Check sheet for the modelled part. Datum: model origin and axes. Units: mm. Face numbers are marked on the shaded views. A direction names the side the tool comes from. Coordinates: 2 decimals unless noted, no trailing zeros. Loops run counter-clockwise (first coordinate to the right, second up) from the corner with the lowest first, then second, coordinate; pieces in that order, holes last. Notation, with made-up numbers: M -28.75,-38.75 L 21.25,-38.75 A22 cw 21.25,-17.75 Z; hole C -29.5,-27.5 d2. An arc over 180 degrees is marked long. Answer in a Markdown table with one row per item. Add a question column.
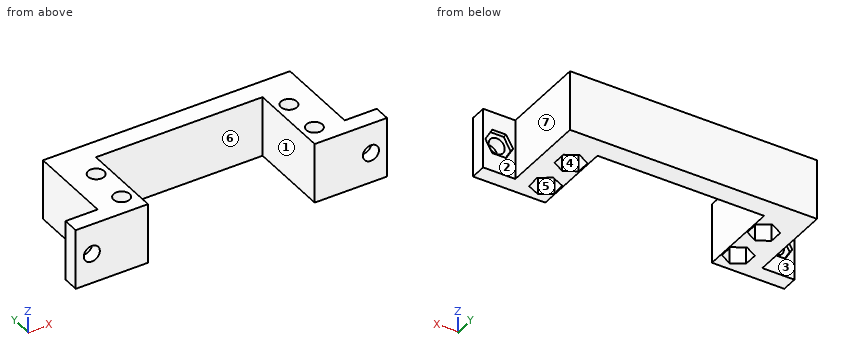
```python
from build123d import *

# Parameters (mm, degrees)
SKETCH1_R           = 2
BOSS_EXTRUDE1_DEPTH = 15
CUT_EXTRUDE1_DEPTH  = 11
CUT_EXTRUDE2_DEPTH  = 1
SKETCH5_R           = 2
CUT_EXTRUDE3_DEPTH  = 4


with BuildPart() as part:
    # Sketch1 → Boss-Extrude1 (new body)
    with BuildSketch(Plane.XY):
        Polygon((0, 0), (0, 20.5), (41.5, 20.5), (41.5, 0), (59.5, 0), (59.5, 4), (51.5, 4), (51.5, 25.5), (-10, 25.5), (-10, 4), (-18, 4), (-18, 0), align=None)
        with Locations((44.75, 5.25)):
            Circle(SKETCH1_R, mode=Mode.SUBTRACT)
        with Locations((44.75, 15.25)):
            Circle(SKETCH1_R, mode=Mode.SUBTRACT)
        with Locations((-3.25, 15.25)):
            Circle(SKETCH1_R, mode=Mode.SUBTRACT)
        with Locations((-3.25, 5.25)):
            Circle(SKETCH1_R, mode=Mode.SUBTRACT)
    extrude(amount=BOSS_EXTRUDE1_DEPTH)

    # Sketch3 → Cut-Extrude1 (cut)
    with BuildSketch(Plane(origin=(0, 0, 0), x_dir=(-1, 0, 0), z_dir=(0, 0, -1))):
        Polygon((3.25, 18.714101615), (0.25, 16.982050808), (0.25, 13.517949192), (3.25, 11.785898385), (6.25, 13.517949192), (6.25, 16.982050808), align=None)
        Polygon((3.25, 8.714101615), (0.25, 6.982050808), (0.25, 3.517949192), (3.25, 1.785898385), (6.25, 3.517949192), (6.25, 6.982050808), align=None)
        Polygon((-44.75, 18.714101615), (-47.75, 16.982050808), (-47.75, 13.517949192), (-44.75, 11.785898385), (-41.75, 13.517949192), (-41.75, 16.982050808), align=None)
        Polygon((-45.037677981, 8.702135771), (-47.883476265, 6.726931446), (-47.595798284, 3.274795675), (-44.462322019, 1.797864229), (-41.616523735, 3.773068554), (-41.904201716, 7.225204325), align=None)
    extrude(amount=-CUT_EXTRUDE1_DEPTH, mode=Mode.SUBTRACT)

    # Sketch4 → Cut-Extrude2 (cut)
    with BuildSketch(Plane(origin=(0, 4, 0), x_dir=(1, 0, 0), z_dir=(0, 1, 0))):
        Polygon((58.964101615, -7.5), (57.232050808, -4.5), (53.767949192, -4.5), (52.035898385, -7.5), (53.767949192, -10.5), (57.232050808, -10.5), align=None)
        Polygon((-17.464101615, -7.5), (-15.732050808, -10.5), (-12.267949192, -10.5), (-10.535898385, -7.5), (-12.267949192, -4.5), (-15.732050808, -4.5), align=None)
    extrude(amount=-CUT_EXTRUDE2_DEPTH, mode=Mode.SUBTRACT)

    # Sketch5 → Cut-Extrude3 (cut)
    with BuildSketch(Plane(origin=(0, 4, 0), x_dir=(1, 0, 0), z_dir=(0, 1, 0))):
        with Locations(Location((55.5, -7.5, 0), (0, 0, 180))):
            Circle(SKETCH5_R)
        with Locations(Location((-14, -7.5, 0), (0, 0, 180))):
            Circle(SKETCH5_R)
    extrude(amount=-CUT_EXTRUDE3_DEPTH, mode=Mode.SUBTRACT)


solid = part.part
```
Q1. Thickness scan on L1, parallel to X at y = 15.25, z = 12; L2, parallel to Y at x = 44.75, z = 13.85; L3, parallel to X at y = 15.25, z = 2.5. Record the ranges inside material, lowest first.
Q2. Cross-section at C-C (x = -14). Record the cut outline in (y, z), plus the area to 3 significant figures.
Q3. Cross-section at D-D (y = 11). Record the cut outline in (x, z), plus the area to 3 significant figures.
Q4. Cross-section at B-B (z = 14). Record the cut outline in (x, y), plus the area to 3 significant figures.
Q5. Mould release check, pull along Y, two halves, no side actions. Record for the marked faces 5, 6 and 7: released by +Y, released by -Y, zero draft, split by the parting line, or undercut.
Q6. Cross-section at A-A (y = 15.25). Record the cut outline in (x, z), plus the area to 3 significant figures.
Q7. Access from +Z, -Z, +X, -X, +Y, -Y to the whole of each face (thin tool, end or side, straight path). Record for the marked faces 1, 2, 3 and 4.
Q8. Go/stop test with flat-tipped pins: pin 1 (1.7 mm diameter, centred on y = 4.5, z = 6, fed in from +X); pin 2 (3.5 mm diameter, centred on x = -3.25, y = 15.25, fed in from -Z); pin 3 (8 mm diameter, centred on y = 8.5, z = 12.5, fed in from +X); pin 4 (6.5 mm diameter, centred on x = -15, z = 11, fed in from +Y). Record where each tip stops, or that it passes through.
Answer key:
| question | item | result |
|---|---|---|
| 1 | L1 | -10 to -5.25, -1.25 to 0, 41.5 to 42.75, 46.75 to 51.5 |
| 1 | L2 | 0 to 3.25, 7.25 to 13.25, 17.25 to 25.5 |
| 1 | L3 | -10 to -6.25, -0.25 to 0, 41.5 to 41.75, 47.75 to 51.5 |
| 2 | outline | M 0,0 L 4,0 L 4,4.5 L 3,4.5 L 3,5.5 L 0,5.5 Z; M 0,9.5 L 3,9.5 L 3,10.5 L 4,10.5 L 4,15 L 0,15 Z |
| 2 | area | 42.0 mm^2 |
| 3 | outline | M -10,0 L 0,0 L 0,15 L -10,15 Z; M 41.5,0 L 51.5,0 L 51.5,15 L 41.5,15 Z |
| 3 | area | 300 mm^2 |
| 4 | outline | M -18,0 L 0,0 L 0,20.5 L 41.5,20.5 L 41.5,0 L 59.5,0 L 59.5,4 L 51.5,4 L 51.5,25.5 L -10,25.5 L -10,4 L -18,4 Z; hole C -3.25,5.25 d4; hole C -3.25,15.25 d4; hole C 44.75,5.25 d4; hole C 44.75,15.25 d4 |
| 4 | area | 731 mm^2 |
| 5 | face 5 | undercut |
| 5 | face 6 | released by -Y |
| 5 | face 7 | zero draft |
| 6 | outline | M -10,0 L -6.25,0 L -6.25,11 L -5.25,11 L -5.25,15 L -10,15 Z; M -1.25,11 L -0.25,11 L -0.25,0 L 0,0 L 0,15 L -1.25,15 Z; M 41.5,0 L 41.75,0 L 41.75,11 L 42.75,11 L 42.75,15 L 41.5,15 Z; M 46.75,11 L 47.75,11 L 47.75,0 L 51.5,0 L 51.5,15 L 46.75,15 Z |
| 6 | area | 136 mm^2 |
| 7 | face 1 | +Z, -Z, -Y |
| 7 | face 2 | +Z, -Z, +X, +Y |
| 7 | face 3 | +Z, -Z, -X, +Y |
| 7 | face 4 | -Z |
| 8 | pin 1 | x = 59.5 |
| 8 | pin 2 | through |
| 8 | pin 3 | x = 51.5 |
| 8 | pin 4 | y = 4 |
